```python
from build123d import *

# Parameters (mm, degrees)
SKETCH_1_W      = 25
SKETCH_1_H      = 32
EXTRUDE_1_DEPTH = 1
SKETCH_3_R      = 0.25


with BuildPart() as part:
    # 草圖1 → 填料-伸長1 (new body)
    with BuildSketch(Plane.XY):
        Rectangle(SKETCH_1_W, SKETCH_1_H)
    extrude(amount=EXTRUDE_1_DEPTH)

    # 掃出1: sweep along a path in 草圖4
    with BuildLine(Plane(origin=(10.5, 0, 0), x_dir=(0, 0, -1), z_dir=(1, 0, 0))) as sweep_1_path:
        ThreePointArc((-1, 4), (-2.341687605, 6.5), (-1, 9))
    # 草圖3 → 掃出1 (sweep)
    with BuildSketch(Plane.XY.offset(1)):
        with Locations((10.5, 4)):
            Circle(SKETCH_3_R)
    sweep(path=sweep_1_path.line)


solid = part.part
```
Geometry check sheet. Reference: the model listing, model coordinates, mm. Give positions to 0.01 mm unless a question says otherwise; leave off trailing zeros. Order: outer loops, then holes, each group sorted by start corner. A loop starts at its lowest first (then second) coordinate and runs counter-clockwise, first axis right, second up. Notation, with made-up numbers: (22, 84) - (78, 84) arc R18 cw to (78, 118) - close; hole circle Ø8 at (-8, 8.25). An arc over 180 degrees is marked (long way). Answer in a Markdown table with one row per item. Add a question column.
Q1. Cross-section at B-B, the plane y = 11. Enter the section's corners in (x, z), then the cut area to 3 significant figures.
Q2. Gauge pin test, flat end, axial feed: pin 1 (10 mm diameter, centred on x = -6.5, y = -10.5, fed in from +Z). Record the tip position at first contact, or that the pin passes through.
Q3. Material ranges on probe 1 along Z at (x, y) = (7.25, 0.5); probe 2 along X at (y, z) = (9, 1.25), recorded low to high. Write a range as from..to.
Q4. Cross-section at A-A, the plane x = -1.5. Enter the section's corners in (y, z), then the cut area to 3 significant figures.
Q5. Mould release check, pull along Y, two halves, no side actions. Record for faces 1 (the flat face through (-0.2, 16, 0.5)), 2 (the flat face through (0, 0, 0)), 3 (the flat face through (-0.2, -16, 0.5)): pulls with the +Y half, pulls with the -Y half, needs draft (parallel to the pull), parting line crosses it, or undercut.
Check values:
| question | item | result |
|---|---|---|
| 1 | outline | (-12.5, 0) - (12.5, 0) - (12.5, 1) - (-12.5, 1) - close |
| 1 | area | 25.0 mm^2 |
| 2 | pin 1 | stops at z = 1 |
| 3 | probe 1 | z = 0..1 |
| 3 | probe 2 | x = 10.32..10.68 |
| 4 | outline | (-16, 0) - (16, 0) - (16, 1) - (-16, 1) - close |
| 4 | area | 32.0 mm^2 |
| 5 | face 1 | pulls with the +Y half |
| 5 | face 2 | needs draft |
| 5 | face 3 | pulls with the -Y half |
